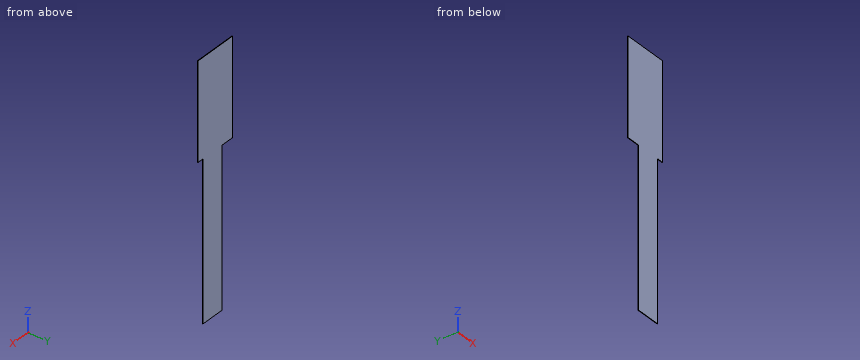
Autodesk Inventor part; units mm, degrees
ref_plane "YZ Plane" through (0, 0, 0) normal (1, 0, 0) x (0, 1, 0)
ref_plane "XZ Plane" through (0, 0, 0) normal (0, 1, 0) x (-1, 0, 0)
ref_plane "XY Plane" through (0, 0, 0) normal (0, 0, 1) x (1, 0, 0)
sketch "Sketch1" plane through (0, 0, 0) normal (0, 1, 0) x (-1, 0, 0)
  line L0 (35, -525) -> (-65, -525)
  line L1 (-90, 125) -> (-90, 525)
  line L2 (-90, 525) -> (90, 525)
  line L3 (-65, -525) -> (-65, 125)
  line L4 (-65, 125) -> (-90, 125)
  line L5 (0, 525) -> (0, -525)
  line L6 (35, -525) -> (35, 125)
  line L7 (35, 125) -> (90, 125)
  line L8 (90, 525) -> (90, 125)
  line L9 (35, 0) -> (-65, 0)
  point P0 (0, 0)
  dimension "d2" = 650
  dimension "d6" = 1050
  dimension "d7" = 180
  dimension "d8" = 55
  dimension "d9" = 155
extrude "Extrusion1" add sketch "Sketch1" along normal blind 2
properties part number "La" material "LCP Plastic"
Geometry check sheet. Reference: the model listing, model coordinates, mm. Coordinates: 2 decimals unless noted, no trailing zeros. Order: outer loops, then holes, each group sorted by start corner. A loop starts at its lowest first (then second) coordinate and runs counter-clockwise, first axis right, second up. Notation, with made-up numbers: (10, 71.5) - (59, 71.5) arc R20 cw to (59, 105.5) - close; hole circle Ø8 at (-18.5, -23). An arc over 180 degrees is marked (long way). Use one line per item in the form item = value.
1. Section check B-B (x = -54). Record the boundary of the cut face in (y, z).
Here are the results:
outline = (0, 125) - (2, 125) - (2, 525) - (0, 525) - close
2. Section check A-A (y = 1.6). Record the boundary of the cut face in (x, z), then the cut area to 3 significant figures.
Here are the results:
outline = (-90, 125) - (-35, 125) - (-35, -525) - (65, -525) - (65, 125) - (90, 125) - (90, 525) - (-90, 525) - close
area = 137,000 mm²
3. Section check C-C (z = -74). Record the boundary of the cut face in (x, y).
Here are the results:
outline = (-35, 0) - (65, 0) - (65, 2) - (-35, 2) - close
4. Gauge pin test, flat ends, axial feed: pin 1 (1 mm diameter, centred on x = 76.5, y = 1.5, fed in from -Z); pin 2 (1 mm diameter, centred on y = 1, z = -197.5, fed in from +X); pin 3 (0.6 mm diameter, centred on y = 1, z = -284.5, fed in from -X). Record the tip position at first contact, or that the pin passes through.
Here are the results:
pin_1 = 125
pin_2 = 65
pin_3 = -35
5. Scan lines: line 1 (X direction, y = 1.9, z = 113); line 2 (Z direction, x = 76, y = 0.3). Record each from-to range of solid material in increasing order.
Here are the results:
line_1 = -35 to 65
line_2 = 125 to 525
